Source: CAD feature listing. Evaluate the final solid. Frame: model axes, mm. Face numbers are marked on the shaded views. A direction names the side the tool comes from. Coordinates: 2 decimals unless noted, no trailing zeros. Loops run counter-clockwise (first coordinate to the right, second up) from the corner with the lowest first, then second, coordinate; pieces in that order, holes last. Notation, with made-up numbers: (45.5, 46) - (102.5, 46) arc R22 ccw to (102.5, 65) - close; hole circle Ø10 at (33.5, -19.5). An arc over 180 degrees is marked (long way). Use CSV: the item, a comma, the result in double quotes. Start each with the question number.
```python
from build123d import *

# Parameters (mm, degrees)
SKETCH1_W           = 24
SKETCH1_H           = 14.5
BOSS_EXTRUDE1_DEPTH = 18
SKETCH2_R           = 1.6
CUT_EXTRUDE1_DEPTH  = 19
SKETCH3_R           = 1.6
CUT_EXTRUDE2_DEPTH  = 25.5
SKETCH4_R           = 3
CUT_EXTRUDE3_DEPTH  = 3.5
CUT_EXTRUDE4_DEPTH  = 3.5
FILLET1_R           = 1
CUT_EXTRUDE5_DEPTH  = 2.6


with BuildPart() as part:
    # Sketch1 → Boss-Extrude1 (new body)
    with BuildSketch(Plane(origin=(0, 0, 0), x_dir=(1, 0, 0), z_dir=(0, 1, 0))):
        with BuildLine():
            Line((0, 0), (30, 0))
            Line((30, 0), (30, 7.25))
            ThreePointArc((30, 7.25), (35, 12.25), (30, 17.25))
            Line((30, 17.25), (30, 24.5))
            Line((30, 24.5), (0, 24.5))
            Line((0, 24.5), (0, 17.25))
            ThreePointArc((0, 17.25), (-5, 12.25), (0, 7.25))
            Line((0, 7.25), (0, 0))
        make_face()
        with Locations((15, 12.25)):
            Rectangle(SKETCH1_W, SKETCH1_H, mode=Mode.SUBTRACT)
    extrude(amount=BOSS_EXTRUDE1_DEPTH)

    # Sketch2 → Cut-Extrude1 (cut, through all)
    with BuildSketch(Plane.XZ):
        with Locations((31, -12.25)):
            Circle(SKETCH2_R)
        with Locations((-1, -12.25)):
            Circle(SKETCH2_R)
    extrude(amount=-CUT_EXTRUDE1_DEPTH, mode=Mode.SUBTRACT)

    # Sketch3 → Cut-Extrude2 (cut, through all)
    with BuildSketch(Plane(origin=(0, 0, -24.5), x_dir=(-1, 0, 0), z_dir=(0, 0, -1))):
        with Locations((-15, 9)):
            Circle(SKETCH3_R)
    extrude(amount=-CUT_EXTRUDE2_DEPTH, mode=Mode.SUBTRACT)

    # Sketch4 → Cut-Extrude3 (cut)
    with BuildSketch(Plane.XY):
        with Locations((15, 9)):
            Circle(SKETCH4_R)
    extrude(amount=-CUT_EXTRUDE3_DEPTH, mode=Mode.SUBTRACT)

    # Sketch5 → Cut-Extrude4 (cut)
    with BuildSketch(Plane(origin=(0, 0, -24.5), x_dir=(-1, 0, 0), z_dir=(0, 0, -1))):
        Polygon((-12.228718708, 7.4), (-12.228718708, 10.6), (-15, 12.2), (-17.771281292, 10.6), (-17.771281292, 7.4), (-15, 5.8), align=None)
    extrude(amount=-CUT_EXTRUDE4_DEPTH, mode=Mode.SUBTRACT)

    # Fillet1
    fillet1_edges = [part.edges().sort_by_distance(p)[0] for p in [
        (0, 9, -24.5),
        (30, 9, -24.5),
        (30, 9, 0),
        (0, 9, 0),
        (27, 9, -5),
        (27, 9, -19.5),
        (3, 9, -19.5),
        (3, 9, -5),
    ]]
    fillet(fillet1_edges, radius=FILLET1_R)

    # Sketch6 → Cut-Extrude5 (cut)
    with BuildSketch(Plane(origin=(0, 2.46, 0), x_dir=(-1, 0, 0), z_dir=(0, -1, 0))):
        Polygon((-32.6, 15.021281292), (-42.6, 15.021281292), (-42.6, 9.478718708), (-32.6, 9.478718708), (-29.4, 9.478718708), (-27.8, 12.25), (-29.4, 15.021281292), align=None)
        Polygon((-0.6, 15.021281292), (2.6, 15.021281292), (12.6, 15.021281292), (12.6, 9.478718708), (2.6, 9.478718708), (-0.6, 9.478718708), (-2.2, 12.25), align=None)
    extrude(amount=-CUT_EXTRUDE5_DEPTH, mode=Mode.SUBTRACT)


solid = part.part
```
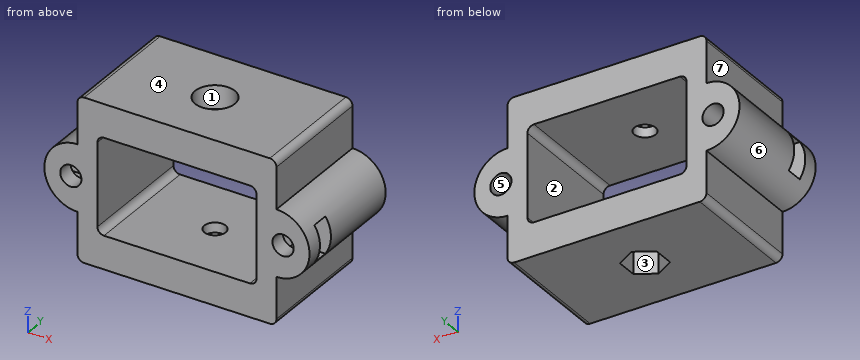
(1) Ray query, line 1 (Z direction, x = 22.5, y = 6.25); line 2 (Y direction, x = 15, z = -1.9); line 3 (Y direction, x = 15, z = -20.5). Return the intervals inside material, ascending. Write a range as [from, to].
(2) Pin query (flat end, axial travel): pin 1 Ø5 at (y, z) = (8.5, -20) entering from +X; pin 2 Ø2.5 at (x, z) = (-1, -12.25) entering from +Y; pin 3 Ø0.8 at (x, y) = (-1, 3.5) entering from -Z; pin 4 Ø5 at (y, z) = (12, -7) entering from +X. Return the tip coordinate at first contact, or that it passes through.
(3) Draft query along Z for the marked faces 4, 5, 6 and 7. Return one class per face: released by +Z, released by -Z, zero draft, split by the parting line, or undercut.
(4) Section D-D on z = -16.5. Output: boundary loops of the cut face in (x, y).
(5) Section C-C on z = -2.75. Output: boundary loops of the cut face in (x, y).
(6) Reachability of the marked faces 1, 2 and 3 from +Z, -Z, +X, -X, +Y, -Y: full face, straight path, thin tool, end or side. Return the list, or none.
(7) Section A-A on x = 9. Output: boundary loops of the cut face in (y, z), plus the area to 3 significant figures.
(8) Section B-B on y = 13.5. Output: boundary loops of the cut face in (x, z).
Solution:
1,line 1,"z = [-24.5, -19.5], [-5, 0]"
1,line 2,"y = [0, 6], [12, 18]"
1,line 3,"y = [0, 7.4], [10.6, 18]"
2,pin 1,"stops at x = 30"
2,pin 2,"passes through"
2,pin 3,"stops at z = -17.21"
2,pin 4,"stops at x = 34.18"
3,face 4,"released by +Z"
3,face 5,"undercut"
3,face 6,"split by the parting line"
3,face 7,"zero draft"
4,outline,"(-2.63, 0) - (3, 0) - (3, 18) - (-2.63, 18) - close; (27, 0) - (32.63, 0) - (32.63, 18) - (27, 18) - close"
5,outline,"(0, 0) - (30, 0) - (30, 18) - (0, 18) - close; hole circle Ø6 at (15, 9)"
6,face 1,"+Z"
6,face 2,"+Y, -Y"
6,face 3,"-Z"
7,outline,"(0, -24.5) - (18, -24.5) - (18, -19.5) - (0, -19.5) - close; (0, -5) - (18, -5) - (18, 0) - (0, 0) - close"
7,area,"180 mm²"
8,outline,"(0, -23.5) arc R1 ccw to (1, -24.5) - (29, -24.5) arc R1 ccw to (30, -23.5) - (30, -17.25) arc R5 ccw to (30, -7.25) - (30, -1) arc R1 ccw to (29, 0) - (1, 0) arc R1 ccw to (0, -1) - (0, -7.25) arc R5 ccw to (0, -17.25) - close; hole circle Ø3.2 at (-1, -12.25); hole (3, -18.5) arc R1 ccw to (4, -19.5) - (26, -19.5) arc R1 ccw to (27, -18.5) - (27, -6) arc R1 ccw to (26, -5) - (4, -5) arc R1 ccw to (3, -6) - close; hole circle Ø3.2 at (31, -12.25)"
